Part model, mm, in its own coordinate system. A direction names the side the tool comes from. Give positions to 0.01 mm unless a question says otherwise; leave off trailing zeros. Write each loop counter-clockwise with the first axis right and the second up, starting at its lowest first coordinate (ties: lowest second). Pieces come first, ordered by that corner, then holes. Notation, with made-up numbers: M -19.5,71 L 36.5,71 A21 ccw 36.5,80 Z; hole C 53.25,12.25 d6. An arc over 180 degrees is marked long. Answer as CSV lines item,"result". Start each with the question number.
Item 1: Band-saw the part on B-B, the plane y = 0. List the corners of the cut face in (x, z), then the cut area to 3 significant figures.
Item 2: Band-saw the part on D-D, the plane z = 32.5. List the corners of the cut face in (x, y).
Item 3: Band-saw the part on A-A, the plane y = 5. List the corners of the cut face in (x, z), then the cut area to 3 significant figures.
Item 4: Wall check: L1, parallel to Z at x = 147.85, y = 10; L2, parallel to Z at x = 146.9, y = 9; L3, parallel to Z at x = 148.2, y = -5. Give the ranges that are in metal, low to high. Write a range as from..to.
Item 5: Band-saw the part on C-C, the plane x = 147.75. Count the separate pieces of the cut face and the enclosed holes in it, then the cut area to 3 significant figures.
Item 6: 3-axis set-ups, long thin cutter, end or side, ignore diameter. For faces 4 (the flat face through (147, 20, 17)), 5 (the flat face through (147, 0, 33.2)): which of +Z, -Z, +X, -X, +Y, -Y reach the whole face in a straight line?
Item 7: Two-plate mould, pull along Z, no slides. Class faces 1 (the cylindrical face through (147.48, 18.95, -2.5)), 2 (the flat face through (147, 0, -0.2)), 3 (the flat face through (147, -20, 16)): +Z half, -Z half, draft (parallel to the pull), parting line (faces both ways), or undercut.
from build123d import *

# Parameters (mm, degrees)
PAD008_DEPTH    = 3
SKETCH034_R     = 1.6
SKETCH034_W     = 5.2
SKETCH034_H     = 3.2
POCKET021_DEPTH = 116.297072
SKETCH035_R     = 1.9
POCKET022_DEPTH = 3.001


with BuildPart() as part:
    # Sketch033 → Pad008 (new body)
    with BuildSketch(Plane.YZ):
        with BuildLine():
            Line((-16.5, 20), (16.5, 20))
            ThreePointArc((20, 16.5), (18.974874, 18.974874), (16.5, 20))
            Line((20, 16.5), (20, -16.5))
            ThreePointArc((16.5, -20), (18.974874, -18.974874), (20, -16.5))
            Line((16.5, -20), (-16.5, -20))
            ThreePointArc((-20, -16.5), (-18.974874, -18.974874), (-16.5, -20))
            Line((-20, -16.5), (-20, 16.5))
            ThreePointArc((-16.5, 20), (-18.974874, 18.974874), (-20, 16.5))
        make_face()
    extrude(amount=PAD008_DEPTH)

    # Sketch034 → Pocket021 (cut, through all)
    with BuildSketch(Plane.YZ):
        with Locations((-10, 15.1)):
            Circle(SKETCH034_R)
        with Locations((10, 15.1)):
            Circle(SKETCH034_R)
        with Locations((0, 15.1)):
            Rectangle(SKETCH034_W, SKETCH034_H)
    pocket021 = extrude(amount=POCKET021_DEPTH, mode=Mode.SUBTRACT)

    # Mirrored019: Pocket021 across Sketch034 H_Axis
    add(pocket021.mirror(Plane.XY), mode=Mode.SUBTRACT)

    # Sketch035 → Pocket022 (cut, through all)
    with BuildSketch(Plane.YZ):
        with Locations((-5, 0)):
            Circle(SKETCH035_R)
        with Locations((5, 0)):
            Circle(SKETCH035_R)
    extrude(amount=POCKET022_DEPTH, mode=Mode.SUBTRACT)


with BuildPart() as part_1:
    # Body006 placement: moved
    add(part.part.moved(Location((146, 0, 16.5))))


solid = part_1.part
Output:
1,outline,"M 146,-3.5 L 149,-3.5 L 149,-0.2 L 146,-0.2 Z; M 146,3 L 149,3 L 149,30 L 146,30 Z; M 146,33.2 L 149,33.2 L 149,36.5 L 146,36.5 Z"
1,area,"101 mm²"
2,outline,"M 146,-20 L 149,-20 L 149,-11.32 L 146,-11.32 Z; M 146,-8.68 L 149,-8.68 L 149,-2.6 L 146,-2.6 Z; M 146,2.6 L 149,2.6 L 149,8.68 L 146,8.68 Z; M 146,11.32 L 149,11.32 L 149,20 L 146,20 Z"
3,outline,"M 146,-3.5 L 149,-3.5 L 149,14.6 L 146,14.6 Z; M 146,18.4 L 149,18.4 L 149,36.5 L 146,36.5 Z"
3,area,"109 mm²"
4,L1,"-3.5..-0.2, 3..30, 33.2..36.5"
4,L2,"-3.5..0.15, 2.65..30.35, 32.85..36.5"
4,L3,"-3.5..14.6, 18.4..36.5"
5,separate pieces,"1"
5,enclosed holes,"8"
5,area,"1,500 mm²"
6,face 4,"+Z, -Z, +X, -X, +Y"
6,face 5,"+X, -X"
7,face 1,"-Z half"
7,face 2,"undercut"
7,face 3,"draft"
